```python
from build123d import *

# Parameters (mm, degrees)
CUT_EXTRUDE3_DEPTH      = 10
CUT_EXTRUDE3_DEPTH_BACK = 10
SKETCH3_R               = 1
CUT_EXTRUDE2_DEPTH      = 8
CHAMFER1_SIZE           = 1


with BuildPart() as part:
    # Sketch4 for Loft1 → Loft1 section 0
    with BuildSketch(Plane(origin=(0, 0, 0), x_dir=(1, 0, 0), z_dir=(0, 1, 0))):
        with BuildLine():
            # circular arc as an exact rational Bezier (weights 1, cos(half-angle), 1)
            Bezier((-1.237436867, -1.237436867), (0, -2.474873734), (1.237436867, -1.237436867), weights=[1, 0.707106781, 1])
            Bezier((1.237436867, -1.237436867), (2.474873734, 0), (1.237436867, 1.237436867), weights=[1, 0.707106781, 1])
            Bezier((1.237436867, 1.237436867), (0, 2.474873734), (-1.237436867, 1.237436867), weights=[1, 0.707106781, 1])
            Bezier((-1.237436867, 1.237436867), (-2.474873734, 0), (-1.237436867, -1.237436867), weights=[1, 0.707106781, 1])
        make_face()
    # Sketch1 → Loft1 section 1
    with BuildSketch(Plane(origin=(0, 14.5, 0), x_dir=(1, 0, 0), z_dir=(0, 1, 0))):
        with BuildLine():
            Line((-2.5, -2.5), (2.5, -2.5))
            Line((2.5, -2.5), (2.5, 2.5))
            Line((2.5, 2.5), (-2.5, 2.5))
            Line((-2.5, 2.5), (-2.5, -2.5))
        make_face()
    loft()

    # Sketch8 → Cut-Extrude3 (cut, two sides: drawn at the far end of the back side and taken through both)
    with BuildSketch(Plane.XY.offset(-CUT_EXTRUDE3_DEPTH_BACK)):
        Polygon((-0.25, 13.25), (-1.5, 13.25), (-1.5, 11), (2.195243382, 11), (3.151773284, 11), (3.151773284, 14.772897757), (-0.25, 14.772897757), align=None)
    extrude(amount=CUT_EXTRUDE3_DEPTH + CUT_EXTRUDE3_DEPTH_BACK, mode=Mode.SUBTRACT)

    # Sketch3 → Cut-Extrude2 (cut)
    with BuildSketch(Plane.XZ):
        with Locations(Location((0, 0, 0), (0, 0, 270))):
            Circle(SKETCH3_R)
    extrude(amount=-CUT_EXTRUDE2_DEPTH, mode=Mode.SUBTRACT)

    # Chamfer1
    chamfer1_edges = [part.edges().sort_by_distance(p)[0] for p in [
        (0, 8, 1),
    ]]
    chamfer(chamfer1_edges, length=CHAMFER1_SIZE)


solid = part.part
```
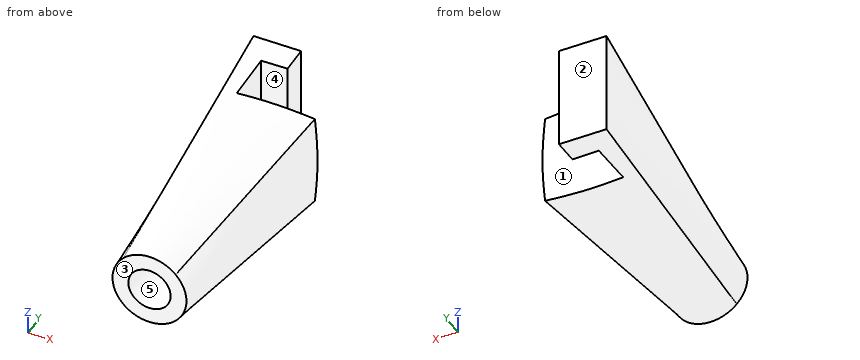
Read the model definition and answer for the solid it produces. Units are mm, in the model's axes. Face numbers are marked on the shaded views. A direction names the side the tool comes from. Coordinates: 2 decimals unless noted, no trailing zeros. Answer as a JSON object with one key per item and string values. Group by question number.
1. Consider L1, parallel to Y at x = 0.1, z = 1.35; L2, parallel to Y at x = -1.4, z = -0.2; L3, parallel to X at y = 7.75, z = 0. Determine where each line is inside the solid, lowest interval first. Write a range as [from, to].
2. Which of the six approach directions +Z, -Z, +X, -X, +Y, -Y give full straight-line access (tool end or side, diameter ignored) to the marked faces 4 and 5?
3. Each of these flat-tipped pins is pushed along its axis until it touches: P1, Ø1.1, axis at y = 11.5, z = -1, coming from the +X side; P2, Ø1, axis at x = 1, y = 12.5, coming from the +Z side; P3, Ø0.6, axis at y = 14, z = -0.5, coming from the +X side. Where does it stop, or does it pass through?
4. The mould has two halves that part along Y. Classify the marked faces 1, 2 and 3: +Y half, -Y half, draft (parallel to the pull), parting line (faces both ways), or undercut.
Worked out:
{
 "1": {"L1": "y = [0, 11]", "L2": "y = [0, 11], [13.25, 14.5]", "L3": "x = [-2.15, -0.25], [0.25, 2.15]"},
 "2": {"face 4": "+Z, -Z, +X", "face 5": "-Y"},
 "3": {"P1": "stops at x = 2.3", "P2": "passes through", "P3": "stops at x = -0.25"},
 "4": {"face 1": "undercut", "face 2": "+Y half", "face 3": "-Y half"}
}
